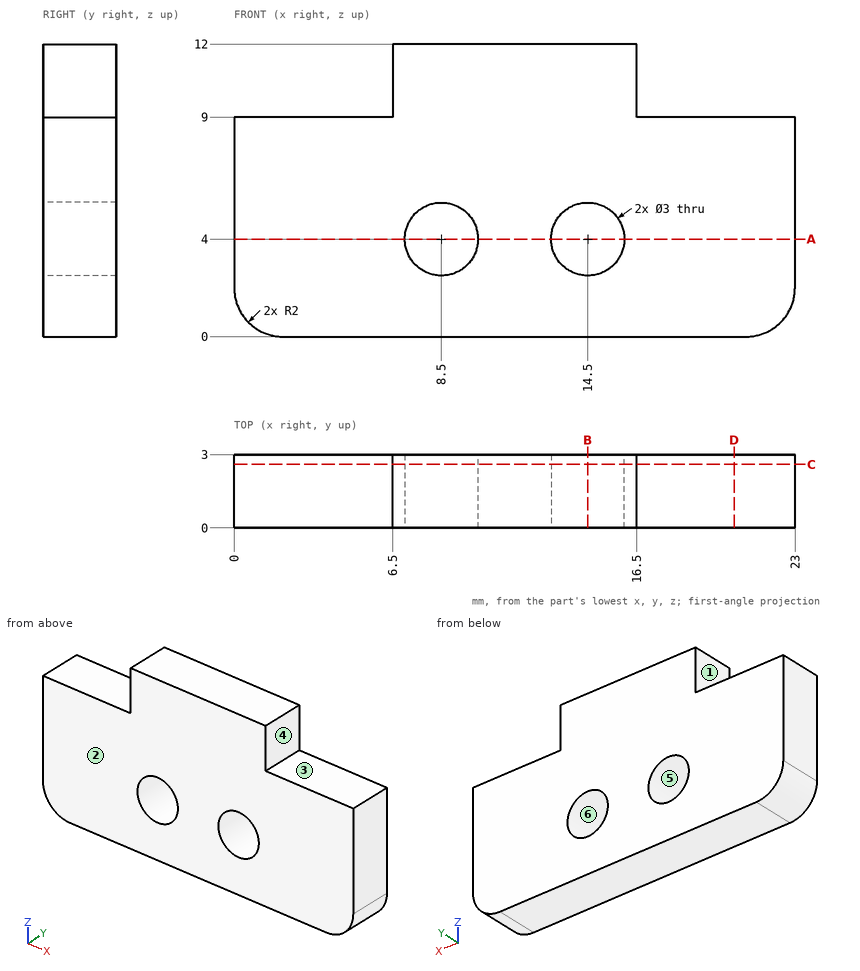
The figure shows three views and two pictorial views of one solid part (mm, origin at its lowest corner). Answer the questions. A direction names the side the tool comes from. Coordinates: 2 decimals unless noted, no trailing zeros. Order: outer loops, then holes, each group sorted by start corner. A loop starts at its lowest first (then second) coordinate and runs counter-clockwise, first axis right, second up. Notation, with made-up numbers: (-5.5, -17.5) - (20.5, -17.5) arc R22 cw to (20.5, 18.5) - close; hole circle Ø10 at (38, -28). An arc over 180 degrees is marked (long way). Answer as a JSON object with one key per item and string values.
1. Each of these flat-tipped pins is pushed along its axis until it touches: P1, Ø1.5, axis at x = 21, y = 2, coming from the +Z side; P2, Ø1.8, axis at x = 8.5, z = 4, coming from the +Y side. Where does it stop, or does it pass through?
Output values:
{"P1": "stops at z = 9", "P2": "passes through"}
2. Consider line 1 (X direction, y = 1.8, z = 4); line 2 (Z direction, x = 14.5, y = 1.05); line 3 (Z direction, x = 20.5, y = 2.6). Determine where each line is inside the solid, lowest interval first.
Output values:
{"line 1": "x = 0 to 7, 10 to 13, 16 to 23", "line 2": "z = 0 to 2.5, 5.5 to 12", "line 3": "z = 0 to 9"}
3. Find section D-D on x = 20.5. Determine the outline of the cut face in (y, z), plus the area to 3 significant figures.
Output values:
{"outline": "(0, 0) - (3, 0) - (3, 9) - (0, 9) - close", "area": "27.0 mm²"}
4. Find section B-B on x = 14.5. Determine the outline of the cut face in (y, z), plus the area to 3 significant figures.
Output values:
{"outline": "(0, 0) - (3, 0) - (3, 2.5) - (0, 2.5) - close; (0, 5.5) - (3, 5.5) - (3, 12) - (0, 12) - close", "area": "27.0 mm²"}
5. A tool of negligible diameter and unlimited length cuts with its end or side. For the marked faces 1 and 2, from which of +Z, -Z, +X, -X, +Y, -Y can it reach the whole face along a straight path? Write none if from no direction.
Output values:
{"face 1": "+Z, -X, +Y, -Y", "face 2": "+Z, -Z, +X, -X, -Y"}
6. Find section C-C on y = 2.6. Determine the outline of the cut face in (x, z), plus the area to 3 significant figures.
Output values:
{"outline": "(0, 2) arc R2 ccw to (2, 0) - (21, 0) arc R2 ccw to (23, 2) - (23, 9) - (16.5, 9) - (16.5, 12) - (6.5, 12) - (6.5, 9) - (0, 9) - close; hole circle Ø3 at (8.5, 4); hole circle Ø3 at (14.5, 4)", "area": "221 mm²"}
7. Find section A-A on z = 4. Determine the outline of the cut face in (x, y), plus the area to 3 significant figures.
Output values:
{"outline": "(0, 0) - (7, 0) - (7, 3) - (0, 3) - close; (10, 0) - (13, 0) - (13, 3) - (10, 3) - close; (16, 0) - (23, 0) - (23, 3) - (16, 3) - close", "area": "51.0 mm²"}
8. The mould has two halves that part along Z. Classify the marked faces 3, 4, 5 and 6: +Z half, -Z half, draft (parallel to the pull), parting line (faces both ways), or undercut.
Output values:
{"face 3": "+Z half", "face 4": "draft", "face 5": "undercut", "face 6": "undercut"}
